from build123d import *

# Parameters (mm, degrees)
F0_W     = 20
F0_H     = 31
F1_DEPTH = 34
F2_W     = 20
F2_H     = 5
F3_DEPTH = 20
F4_W     = 20
F4_H     = 10
F5_DEPTH = 30
F6_W     = 20
F6_H     = 10
F7_DEPTH = 30
F9_DEPTH = 20


with BuildPart() as f1:
    # F0 (on Top) → F1 (new body)
    with BuildSketch(Plane.XY):
        with Locations((10, 15.5)):
            Rectangle(F0_W, F0_H)
    extrude(amount=F1_DEPTH)

    # F2 (on face) → F3 (join)
    with BuildSketch(Plane.XY.offset(34)):
        with Locations((10, 28.5)):
            Rectangle(F2_W, F2_H)
        with Locations((10, 2.5)):
            Rectangle(F2_W, F2_H)
    extrude(amount=F3_DEPTH)

    # F4 (on face) → F5 (join)
    with BuildSketch(Plane.XZ):
        with Locations((10, 5)):
            Rectangle(F4_W, F4_H)
    extrude(amount=F5_DEPTH)

    # F6 (on face) → F7 (join)
    with BuildSketch(Plane(origin=(0, 31, 0), x_dir=(-1, 0, 0), z_dir=(0, 1, 0))):
        with Locations((-10, 5)):
            Rectangle(F6_W, F6_H)
    extrude(amount=F7_DEPTH)

    # F8 (on face) → F9 (cut)
    with BuildSketch(Plane.YZ.offset(20)):
        Polygon((-30, 1), (0, 10), (-30, 10), align=None)
        Polygon((31, 10), (61, 1), (61, 10), align=None)
    extrude(amount=-F9_DEPTH, mode=Mode.SUBTRACT)


solid = f1.part
Input: part model. Units: mm. Frame: model coordinates. A direction names the side the tool comes from. Round coordinates to 2 decimals unless told otherwise and drop trailing zeros. Loops run counter-clockwise (first coordinate to the right, second up) from the corner with the lowest first, then second, coordinate; pieces in that order, holes last. Notation, with made-up numbers: (-38.5, 80.25) -> (2.5, 80.25) arc R12 ccw to (2.5, 96.25) -> close; hole circle Ø7 at (52.25, 68.25). An arc over 180 degrees is marked (long way). Answer as a JSON object with one key per item and string values. Group by question number.
1) Reachability of faces 4 (the flat face through (10, 31, 32)), 5 (the flat face through (10.14, -15.21, 5.437)), 6 (the flat face through (10, 16, 34)) from +Z, -Z, +X, -X, +Y, -Y: full face, straight path, thin tool, end or side. Return the list, or none.
2) Section query A-A on z = 42.5. Output: boundary loops of the cut face in (x, y), plus the area to 3 significant figures.
3) Draft query along Y for faces 1 (the flat face through (10, 0, 32)), 2 (the flat face through (0, 15, 15)), 3 (the flat face through (10, 26, 44)). Return one class per face: +Y half, -Y half, draft (parallel to the pull), parting line (faces both ways), or undercut.
4) Section query C-C on y = 39. Output: boundary loops of the cut face in (x, z), plus the area to 3 significant figures.
5) Pin query (flat end, axial travel): pin 1 (10 mm diameter, centred on x = 10, z = 25.5, fed in from +Y); pin 2 (12 mm diameter, centred on x = 13, z = 17.5, fed in from -Y); pin 3 (4 mm diameter, centred on x = 16, y = 35.5, fed in from +Z); pin 4 (1 mm diameter, centred on y = -1, z = 15.5, fed in from +X). Return the tip coordinate at first contact, or that it passes through.
6) Section query B-B on x = 9. Output: boundary loops of the cut face in (y, z).
7) Ray query, L1, parallel to Y at x = 16.25, z = 43; L2, parallel to Z at x = 9, y = 15; L3, parallel to Y at x = 19, z = 32.5. Return the intervals inside material, ascending.
8) Section query D-D on z = 16. Output: boundary loops of the cut face in (x, y).
Reply:
{
 "1": {"face 4": "+Z, +X, -X, +Y", "face 5": "+Z, +X, -X, -Y", "face 6": "+Z, +X, -X"},
 "2": {"outline": "(0, 0) -> (20, 0) -> (20, 5) -> (0, 5) -> close; (0, 26) -> (20, 26) -> (20, 31) -> (0, 31) -> close", "area": "200 mm2"},
 "3": {"face 1": "-Y half", "face 2": "draft", "face 3": "undercut"},
 "4": {"outline": "(0, 0) -> (20, 0) -> (20, 7.6) -> (0, 7.6) -> close", "area": "152 mm2"},
 "5": {"pin 1": "stops at y = 31", "pin 2": "stops at y = 0", "pin 3": "stops at z = 9.25", "pin 4": "passes through"},
 "6": {"outline": "(-30, 0) -> (61, 0) -> (61, 1) -> (31, 10) -> (31, 54) -> (26, 54) -> (26, 34) -> (5, 34) -> (5, 54) -> (0, 54) -> (0, 10) -> (-30, 1) -> close"},
 "7": {"L1": "y = 0 to 5, 26 to 31", "L2": "z = 0 to 34", "L3": "y = 0 to 31"},
 "8": {"outline": "(0, 0) -> (20, 0) -> (20, 31) -> (0, 31) -> close"}
}
